Design review of the part built by this model. Coordinates are the model's own, in mm. A direction names the side the tool comes from. Coordinates: 2 decimals unless noted, no trailing zeros. Loops run counter-clockwise (first coordinate to the right, second up) from the corner with the lowest first, then second, coordinate; pieces in that order, holes last. Notation, with made-up numbers: (-10.5, 52.25) -> (-0.5, 52.25) arc R22 ccw to (-0.5, 71.25) -> close; hole circle Ø8 at (-18, -4). An arc over 180 degrees is marked (long way). Answer in a Markdown table with one row per item.
Autodesk Inventor part; units mm, degrees
ref_plane "YZ Plane" through (0, 0, 0) normal (1, 0, 0) x (0, 1, 0)
ref_plane "XZ Plane" through (0, 0, 0) normal (0, 1, 0) x (-1, 0, 0)
ref_plane "XY Plane" through (0, 0, 0) normal (0, 0, 1) x (1, 0, 0)
sketch "Sketch1" plane through (0, 0, 0) normal (0, 0, 1) x (1, 0, 0)
  line L0 (-114.7642, 55) -> (135.2358, 55)
  line L1 (135.2358, 55) -> (135.2358, -75)
  line L2 (135.2358, -75) -> (-114.7642, -75)
  line L3 (-114.7642, -75) -> (-114.7642, 55)
  point P0 (0, 0)
  dimension "d0" = 250
  dimension "d1" = 130
extrude "Extrusion1" add sketch "Sketch1" along normal blind 10
sketch "Sketch2" plane through (0, 0, 10) normal (0, 0, 1) x (1, 0, 0)
  line L0 (135.2358, 55) -> (-114.7642, 55)
  line L1 (135.2358, -75) -> (135.2358, 55)
  line L2 (-114.7642, 55) -> (135.2358, 55)
  line L3 (135.2358, 55) -> (135.2358, 40)
  line L4 (135.2358, 40) -> (-114.7642, 40)
  line L5 (-114.7642, 40) -> (-114.7642, 55)
  line L6 (-114.7642, -75) -> (135.2358, -75)
  line L7 (135.2358, -75) -> (135.2358, -60)
  line L8 (135.2358, -60) -> (-114.7642, -60)
  line L9 (-114.7642, -60) -> (-114.7642, -75)
  point P0 (0, 0)
  dimension "d4" = 15
  dimension "d5" = 15
extrude "Extrusion2" add sketch "Sketch2" along normal blind 21
sketch "Sketch3" plane through (0, 0, 31) normal (0, 0, 1) x (1, 0, 0)
  line L0 (-114.7642, 55) -> (-114.7642, -75)
  line L1 (135.2358, -60) -> (135.2358, 40)
  line L2 (-114.7642, 55) -> (135.2358, 55)
  line L3 (135.2358, 55) -> (135.2358, 25)
  line L4 (135.2358, 25) -> (-114.7642, 25)
  line L5 (-114.7642, 25) -> (-114.7642, 55)
  line L6 (135.2358, -75) -> (135.2358, -60)
  line L7 (135.2358, -75) -> (-114.7642, -75)
  line L8 (-114.7642, -75) -> (-114.7642, -45)
  line L9 (-114.7642, -45) -> (135.2358, -45)
  line L10 (135.2358, -45) -> (135.2358, -75)
  point P0 (0, 0)
  point P1 (-114.7642, -45)
  dimension "d8" = 30
  dimension "d9" = 30
extrude "Extrusion3" add sketch "Sketch3" along normal blind 10 contours L2 L3 L1 L4 L0 | L9 L1 L6 L7 L0
sketch "Sketch4" plane through (-114.7642, -75, 0) normal (-1, 0, 0) x (0, 0, 1)
  line L0 (7.1242, 110) -> (2.1242, 110)
  line L1 (2.1242, 110) -> (2.1242, 100)
  line L2 (2.1242, 100) -> (7.1242, 100)
  line L3 (7.1242, 100) -> (7.1242, 110)
  line L4 (7.1242, 30) -> (2.1242, 30)
  line L5 (2.1242, 30) -> (2.1242, 20)
  line L6 (2.1242, 20) -> (7.1242, 20)
  line L7 (7.1242, 20) -> (7.1242, 30)
  line L8 (31, 100) -> (41, 100)
  line L9 (31, 30) -> (41, 30)
  point P0 (0, 75)
  dimension "d12" = 5
  dimension "d13" = 10
  dimension "d14" = 10
  dimension "d15" = 0
  dimension "d16" = 0
extrude "Extrusion4" add sketch "Sketch4" along normal blind 20
equation "\"d5\" = d4"
equation "\"d9\" = d8"
properties part number "Part2_with_things"
(1) Take a section at A-A on z = 35.5. Give the boundary of the cut face in (x, y).
Evaluation:
| item | result |
|---|---|
| outline | (-114.76, -75) -> (135.24, -75) -> (135.24, -45) -> (-114.76, -45) -> close; (-114.76, 25) -> (135.24, 25) -> (135.24, 55) -> (-114.76, 55) -> close |
(2) Take a section at D-D on y = 47. Give the boundary of the cut face in (x, z).
Evaluation:
| item | result |
|---|---|
| outline | (-114.76, 0) -> (135.24, 0) -> (135.24, 41) -> (-114.76, 41) -> close |
(3) Take a section at C-C on z = 17. Give the boundary of the cut face in (x, y).
Evaluation:
| item | result |
|---|---|
| outline | (-114.76, -75) -> (135.24, -75) -> (135.24, -60) -> (-114.76, -60) -> close; (-114.76, 40) -> (135.24, 40) -> (135.24, 55) -> (-114.76, 55) -> close |
(4) Take a section at B-B on x = -38.5. Give the boundary of the cut face in (y, z), and give its area (3 significant figures).
Evaluation:
| item | result |
|---|---|
| outline | (-75, 0) -> (55, 0) -> (55, 41) -> (25, 41) -> (25, 31) -> (40, 31) -> (40, 10) -> (-60, 10) -> (-60, 31) -> (-45, 31) -> (-45, 41) -> (-75, 41) -> close |
| area | 2,530 mm² |
(5) Tool access review of faces 4 (the flat face through (8, -45, 36)), 5 (the flat face through (-125, -45, 5)), 6 (the flat face through (-125, -50, 2.124)), 7 (the flat face through (-125, 35, 5)), 8 (the flat face through (12, -60, 20)): name each direction out of +Z, -Z, +X, -X, +Y, -Y from which nothing blocks a thin tool from reaching the whole face with its end or side.
Evaluation:
| item | result |
|---|---|
| face 4 | +Z, +X, -X |
| face 5 | +Z, -Z, -X |
| face 6 | -Z, -X, +Y, -Y |
| face 7 | +Z, -Z, -X, +Y |
| face 8 | +X, -X |
(6) For pin 1 (3 mm diameter, centred on x = -125.5, y = 30, fed in from -Z); pin 2 (1 mm diameter, centred on x = -71, y = 8.5, fed in from +Z); pin 3 (5.5 mm diameter, centred on x = -120.5, z = 5, fed in from +Y), all flat-tipped, find the tip position at first contact; note any pin that passes through.
Evaluation:
| item | result |
|---|---|
| pin 1 | stops at z = 2.12 |
| pin 2 | stops at z = 10 |
| pin 3 | stops at y = 35 |
(7) To check wall thickness, follow probe 1 along Y at (x, z) = (-21, 11); probe 2 along Y at (x, z) = (-21, 38.5); probe 3 along X at (y, z) = (47, 38.5). State the ranges of each line that lie inside material, in increasing order.
Evaluation:
| item | result |
|---|---|
| probe 1 | y = -75 to -60, 40 to 55 |
| probe 2 | y = -75 to -45, 25 to 55 |
| probe 3 | x = -114.76 to 135.24 |
(8) Draft analysis for pull direction Y (two halves, no side actions). For faces 1 (the flat face through (12, -75, 20)), 2 (the flat face through (-125, 30, 7.124)), 3 (the flat face through (8, -9, 10)), state which applies: pulls with the +Y half, pulls with the -Y half, needs draft (parallel to the pull), parting line crosses it, or undercut.
Evaluation:
| item | result |
|---|---|
| face 1 | pulls with the -Y half |
| face 2 | needs draft |
| face 3 | undercut |
